Could you check a few things on this model? Use its own coordinates, in mm. Face numbers are marked on the shaded views. A direction names the side the tool comes from. Give positions to 0.01 mm unless a question says otherwise; leave off trailing zeros. Loops run counter-clockwise (first coordinate to the right, second up) from the corner with the lowest first, then second, coordinate; pieces in that order, holes last. Notation, with made-up numbers: (38, -29.75) -> (61, -29.75) arc R25 cw to (61, -3.75) -> close; hole circle Ø1 at (-18.5, -14.75). An arc over 180 degrees is marked (long way). Put each result on its own line as item: value.
```python
from build123d import *

# Parameters (mm, degrees)
SKETCH2_W            = 41
SKETCH2_H            = 41
SKETCH2_W_2          = 14.993938253
SKETCH2_H_2          = 4.00275912
BOSS_EXTRUDE7_DEPTH  = 23
CUT_EXTRUDE1_DEPTH   = 23
CUT_EXTRUDE3_DEPTH   = 23
SKETCH8_W            = 14.993938253
SKETCH8_H            = 4.00275912
CUT_EXTRUDE4_DEPTH   = 14
SKETCH3_R            = 2
BOSS_EXTRUDE11_DEPTH = 20


with BuildPart() as part:
    # Sketch2 → Boss-Extrude7 (new body)
    with BuildSketch(Plane(origin=(0, 0, 0), x_dir=(1, 0, 0), z_dir=(0, 1, 0))):
        Rectangle(SKETCH2_W, SKETCH2_H)
        with Locations((0.012281963, 22.50137956)):
            Rectangle(SKETCH2_W_2, SKETCH2_H_2)
    extrude(amount=BOSS_EXTRUDE7_DEPTH)

    # Sketch6 → Cut-Extrude1 (cut)
    with BuildSketch(Plane(origin=(0, 0, 0), x_dir=(1, 0, 0), z_dir=(0, 1, 0))):
        Polygon((-20.5, 20.5), (-15.5, 20.5), (-20.5, 15.5), align=None)
    extrude(amount=CUT_EXTRUDE1_DEPTH, mode=Mode.SUBTRACT)

    # Sketch7 → Cut-Extrude3 (cut)
    with BuildSketch(Plane(origin=(0, 0, 0), x_dir=(1, 0, 0), z_dir=(0, 1, 0))):
        Polygon((-20.5, -20.5), (-20.5, -15.5), (-15.5, -20.5), align=None)
        Polygon((20.5, -20.5), (15.5, -20.5), (20.5, -15.5), align=None)
        Polygon((20.5, 20.5), (20.5, 15.5), (15.5, 20.5), align=None)
    extrude(amount=CUT_EXTRUDE3_DEPTH, mode=Mode.SUBTRACT)

    # Sketch8 → Cut-Extrude4 (cut)
    with BuildSketch(Plane(origin=(0, 23, 0), x_dir=(1, 0, 0), z_dir=(0, 1, 0))):
        with Locations((0.012281963, 22.50137956)):
            Rectangle(SKETCH8_W, SKETCH8_H)
    extrude(amount=-CUT_EXTRUDE4_DEPTH, mode=Mode.SUBTRACT)

    # Sketch3 → Boss-Extrude11 (add)
    with BuildSketch(Plane(origin=(0, 23, 0), x_dir=(1, 0, 0), z_dir=(0, 1, 0))):
        Circle(SKETCH3_R)
    extrude(amount=BOSS_EXTRUDE11_DEPTH)


solid = part.part
```
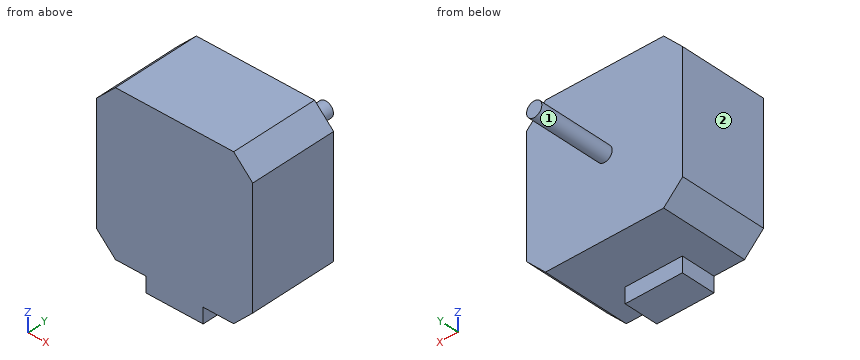
1. If we section it at C-C (z = 0): List the corners of the cut face in (x, y) for me.
Recorded:
outline: (-20.5, 0) -> (20.5, 0) -> (20.5, 23) -> (2, 23) -> (2, 43) -> (-2, 43) -> (-2, 23) -> (-20.5, 23) -> close
2. If we section it at D-D (y = 5): List the corners of the cut face in (x, z) for me, then the cut area to 3 significant figures.
Recorded:
outline: (-20.5, -15.5) -> (-15.5, -20.5) -> (-7.48, -20.5) -> (-7.48, -24.5) -> (7.51, -24.5) -> (7.51, -20.5) -> (15.5, -20.5) -> (20.5, -15.5) -> (20.5, 15.5) -> (15.5, 20.5) -> (-15.5, 20.5) -> (-20.5, 15.5) -> close
area: 1,690 mm^2
3. For the marked faces 1 and 2, which set-ups out of +Z, -Z, +X, -X, +Y, -Y let a thin tool reach every point of the face, with its end or its side?
Recorded:
face 1: +Y
face 2: +Z, -Z, -X, +Y, -Y
4. If we section it at B-B (x = 0): List the corners of the cut face in (y, z) for me.
Recorded:
outline: (0, -24.5) -> (9, -24.5) -> (9, -20.5) -> (23, -20.5) -> (23, -2) -> (43, -2) -> (43, 2) -> (23, 2) -> (23, 20.5) -> (0, 20.5) -> close
5. I need wall thicknesses on line 1 (Y direction, x = 9.5, z = 14); line 2 (X direction, y = 7, z = -21); line 3 (Z direction, x = 7, y = 13.5). Which ranges of each line are inside material? Lowest first, please.
Recorded:
line 1: y = 0 to 23
line 2: x = -7.48 to 7.51
line 3: z = -20.5 to 20.5
6. If we section it at A-A (y = 17): List the corners of the cut face in (x, z) for me, then the cut area to 3 significant figures.
Recorded:
outline: (-20.5, -15.5) -> (-15.5, -20.5) -> (15.5, -20.5) -> (20.5, -15.5) -> (20.5, 15.5) -> (15.5, 20.5) -> (-15.5, 20.5) -> (-20.5, 15.5) -> close
area: 1,630 mm^2
7. I'm going to push flat-ended pins straight in: pin 1 (2 mm diameter, centred on y = 5, z = -23, fed in from +X); pin 2 (3 mm diameter, centred on x = 15, z = 7.5, fed in from +Y); pin 3 (4.5 mm diameter, centred on y = 6.5, z = -23, fed in from -X). Where does each tip first touch, or does it pass through?
Recorded:
pin 1: stops at x = 7.51
pin 2: stops at y = 23
pin 3: stops at x = -7.48
